from build123d import *

# Parameters (mm, degrees)
ESQUISSE1_W        = 20
ESQUISSE1_H        = 3
ESQUISSE1_W_2      = 3
ESQUISSE1_H_2      = 20
BOSS_EXTRU_1_DEPTH = 3


with BuildPart() as part:
    # Esquisse1 → Boss.-Extru.1 (new body)
    with BuildSketch(Plane.XY):
        Polygon((10, -62), (30, -62), (30, -35), (27, -35), (27, -15), (30, -15), (30, 15), (27, 15), (27, 35), (30, 35), (30, 62), (10, 62), (10, 59), (-10, 59), (-10, 62), (-30, 62), (-30, 35), (-27, 35), (-27, 15), (-30, 15), (-30, -15), (-27, -15), (-27, -35), (-30, -35), (-30, -62), (-10, -62), (-10, -59), (10, -59), align=None)
        with Locations((0, 60.5)):
            Rectangle(ESQUISSE1_W, ESQUISSE1_H)
        with Locations((0, 63.5)):
            Rectangle(ESQUISSE1_W, ESQUISSE1_H)
        with Locations((-28.5, 25)):
            Rectangle(ESQUISSE1_W_2, ESQUISSE1_H_2)
        with Locations((-31.5, 25)):
            Rectangle(ESQUISSE1_W_2, ESQUISSE1_H_2)
        with Locations((31.5, 25)):
            Rectangle(ESQUISSE1_W_2, ESQUISSE1_H_2)
        with Locations((28.5, 25)):
            Rectangle(ESQUISSE1_W_2, ESQUISSE1_H_2)
        with Locations((31.5, -25)):
            Rectangle(ESQUISSE1_W_2, ESQUISSE1_H_2)
        with Locations((28.5, -25)):
            Rectangle(ESQUISSE1_W_2, ESQUISSE1_H_2)
        with Locations((0, -60.5)):
            Rectangle(ESQUISSE1_W, ESQUISSE1_H)
        with Locations((0, -63.5)):
            Rectangle(ESQUISSE1_W, ESQUISSE1_H)
        with Locations((-28.5, -25)):
            Rectangle(ESQUISSE1_W_2, ESQUISSE1_H_2)
        with Locations((-31.5, -25)):
            Rectangle(ESQUISSE1_W_2, ESQUISSE1_H_2)
    extrude(amount=BOSS_EXTRU_1_DEPTH)


solid = part.part
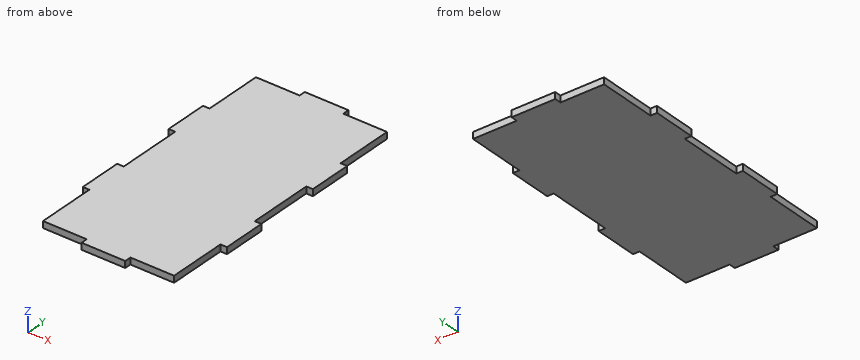
Verification items for the finished model (mm, model axes). Coordinates: 2 decimals unless noted, no trailing zeros. Loops run counter-clockwise (first coordinate to the right, second up) from the corner with the lowest first, then second, coordinate; pieces in that order, holes last. Notation, with made-up numbers: (-18.75, 24) -> (18.25, 24) arc R27 cw to (18.25, 63) -> close; hole circle Ø11 at (62, 82). An arc over 180 degrees is marked (long way). Answer as CSV lines item,"result".
1) Thickness scan on L1, parallel to Y at x = -16, z = 2.05; L2, parallel to X at y = -38.5, z = 2.3. Record the ranges inside material, lowest first. Write a range as from..to.
Found:
L1,"y = -62..62"
L2,"x = -30..30"
2) Depth check by flat-ended pin: pin 1 (0.9 mm diameter, centred on y = -63, z = 2, fed in from -X); pin 2 (1.5 mm diameter, centred on y = 53.5, z = 1, fed in from +X); pin 3 (1.5 mm diameter, centred on x = 16, z = 2, fed in from -Y). Enter the tip coordinate at first touch or a pass-through.
Found:
pin 1,"stops at x = -10"
pin 2,"stops at x = 30"
pin 3,"stops at y = -62"
3) Cross-section at B-B, the plane y = 2. Record the cut outline in (x, z), then the cut area to 3 significant figures.
Found:
outline,"(-30, 0) -> (30, 0) -> (30, 3) -> (-30, 3) -> close"
area,"180 mm2"
4) Cross-section at A-A, the plane z = 2.4. Record the cut outline in (x, y), then the cut area to 3 significant figures.
Found:
outline,"(-33, -35) -> (-30, -35) -> (-30, -62) -> (-10, -62) -> (-10, -65) -> (10, -65) -> (10, -62) -> (30, -62) -> (30, -35) -> (33, -35) -> (33, -15) -> (30, -15) -> (30, 15) -> (33, 15) -> (33, 35) -> (30, 35) -> (30, 62) -> (10, 62) -> (10, 65) -> (-10, 65) -> (-10, 62) -> (-30, 62) -> (-30, 35) -> (-33, 35) -> (-33, 15) -> (-30, 15) -> (-30, -15) -> (-33, -15) -> close"
area,"7,800 mm2"
5) Cross-section at C-C, the plane x = 12.5. Record the cut outline in (y, z).
Found:
outline,"(-62, 0) -> (62, 0) -> (62, 3) -> (-62, 3) -> close"
